For this review, use the dimensioned drawing (mm, ordinates from the lowest corner) and the shaded views. A direction names the side the tool comes from. Coordinates: 2 decimals unless noted, no trailing zeros. Write each loop counter-clockwise with the first axis right and the second up, starting at its lowest first coordinate (ties: lowest second). Pieces come first, ordered by that corner, then holes. Notation, with made-up numbers: M 4,50.25 L 58,50.25 A12 cw 58,62.25 Z; hole C 73,15.25 d11. An arc over 180 degrees is marked long. Return JSON: item names as keys, results as strings.
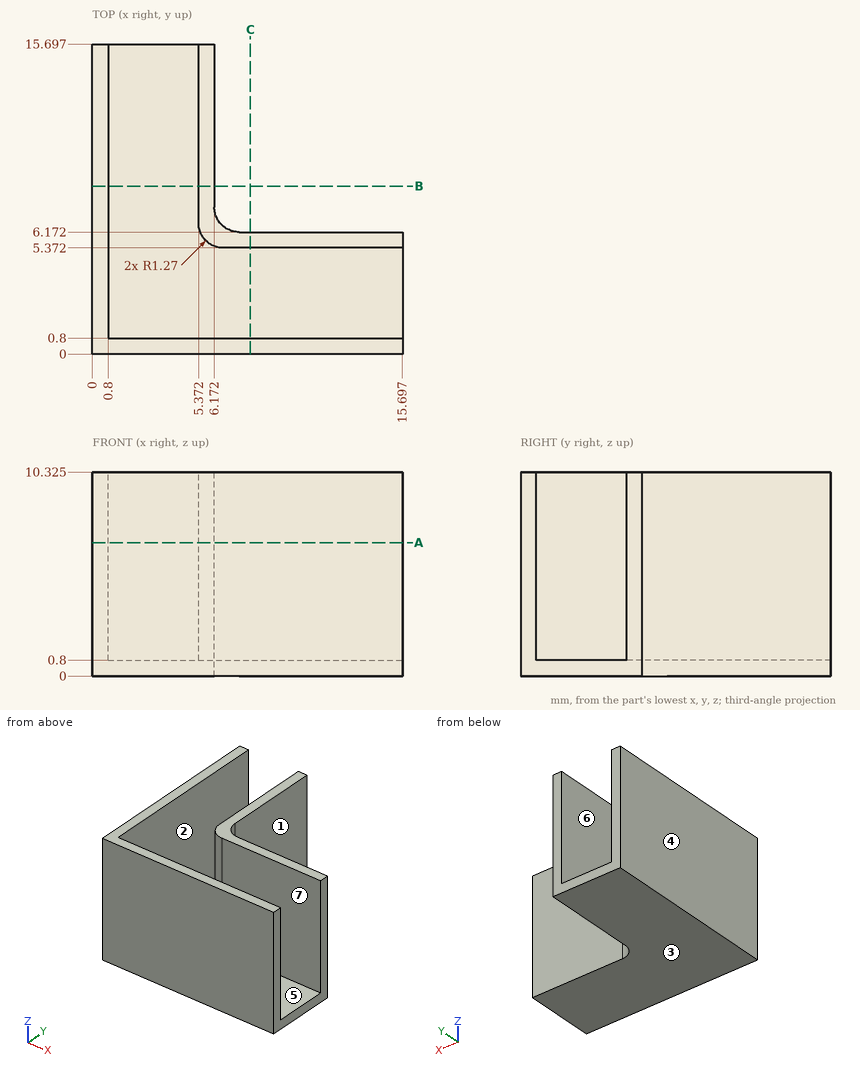
1. For the marked faces 1, 2 and 3, list the 3-axis set-ups (+Z, -Z, +X, -X, +Y, -Y) from which the entire face can be reached by the end or side of a thin tool; tool diameter is ignored.
Checks:
{"face 1": "+Z, -Z, +X, +Y", "face 2": "+Z, +Y", "face 3": "-Z, +X, -X, +Y, -Y"}
2. Clearance check with flat-ended pins moving along their axes: pin 1 Ø5 at (x, z) = (13.5, 1) entering from +Y; pin 2 Ø6 at (y, z) = (13.5, 6) entering from +X; pin 3 Ø6 at (y, z) = (10, 5.5) entering from +X. State where each tip first meets the part, or that it passes through.
Checks:
{"pin 1": "y = 6.17", "pin 2": "x = 6.17", "pin 3": "x = 6.25"}
3. We need section B-B (y = 8.5). State the section outline as (x, z) points (3 decimals).
Checks:
{"outline": "M 0,0 L 6.172,0 L 6.172,10.325 L 5.372,10.325 L 5.372,0.8 L 0.8,0.8 L 0.8,10.325 L 0,10.325 Z"}
4. We need section A-A (z = 6.75). State the section outline as (x, y) points.
Checks:
{"outline": "M 0,0 L 15.7,0 L 15.7,0.8 L 0.8,0.8 L 0.8,15.7 L 0,15.7 Z; M 5.37,6.64 A1.27 ccw 6.64,5.37 L 15.7,5.37 L 15.7,6.17 L 7.44,6.17 A1.27 cw 6.17,7.44 L 6.17,15.7 L 5.37,15.7 Z"}
5. Wall thickness on L1, parallel to X at y = 14.75, z = 9; L2, parallel to Y at x = 5.75, z = 5: over which ranges is each line inside the solid? List them lowest first. Write a range as from..to.
Checks:
{"L1": "0..0.8, 5.37..6.17", "L2": "0..0.8, 5.74..15.7"}
6. Draft analysis for pull direction X (two halves, no side actions). For the marked faces 4, 5, 6 and 7, state which applies: +X half, -X half, draft (parallel to the pull), parting line (faces both ways), or undercut.
Checks:
{"face 4": "-X half", "face 5": "undercut", "face 6": "undercut", "face 7": "draft"}
